Part model, mm, in its own coordinate system. Give positions to 0.01 mm unless a question says otherwise; leave off trailing zeros. Loops run counter-clockwise (first coordinate to the right, second up) from the corner with the lowest first, then second, coordinate; pieces in that order, holes last. Notation, with made-up numbers: (9, 72.25) -> (25, 72.25) arc R22 ccw to (25, 110.25) -> close; hole circle Ø1 at (66, -25.5). An arc over 180 degrees is marked (long way). Write item = value, one per line.
from build123d import *

# Parameters (mm, degrees)
SKETCH1_R           = 1.0922
SKETCH1_R_2         = 2.1
BOSS_EXTRUDE1_DEPTH = 1.5875


with BuildPart() as part:
    # Sketch1 → Boss-Extrude1 (new body)
    with BuildSketch(Plane.XY):
        with BuildLine():
            Line((13.360883802, 35.680481836), (49.041365638, 22.319598034))
            ThreePointArc((49.041365638, 22.319598034), (64.516692787, 0), (49.041365638, -22.319598034))
            Line((49.041365638, -22.319598034), (13.360883802, -35.680481836))
            ThreePointArc((13.360883802, -35.680481836), (-38.1, 0), (13.360883802, 35.680481836))
        make_face()
        with Locations((61.341692787, 0)):
            Circle(SKETCH1_R, mode=Mode.SUBTRACT)
        with Locations((25.4, 27.782025366)):
            Circle(SKETCH1_R, mode=Mode.SUBTRACT)
        with Locations((25.4, -27.782025366)):
            Circle(SKETCH1_R, mode=Mode.SUBTRACT)
        with Locations((-34.925, 0)):
            Circle(SKETCH1_R, mode=Mode.SUBTRACT)
        with Locations((6.35, 0)):
            Circle(SKETCH1_R_2, mode=Mode.SUBTRACT)
        with Locations((-3.175, -5.499261314)):
            Circle(SKETCH1_R_2, mode=Mode.SUBTRACT)
        with Locations((-3.175, 5.499261314)):
            Circle(SKETCH1_R_2, mode=Mode.SUBTRACT)
    extrude(amount=BOSS_EXTRUDE1_DEPTH)


solid = part.part
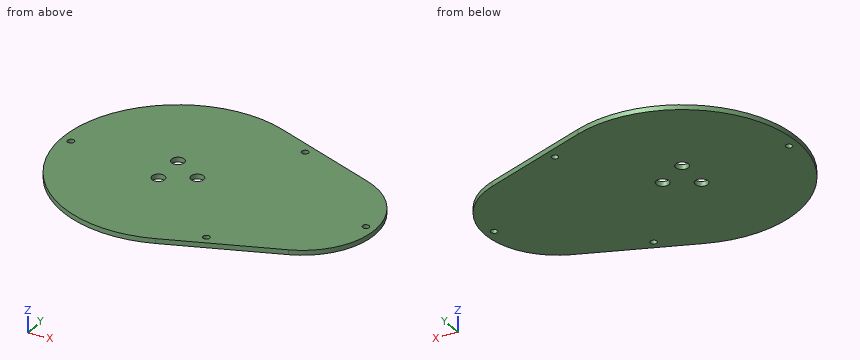
1) Slice it at C-C, the plane z = 0.9. List the corners of the cut face in (x, y) (3 decimals), and give its area (3 significant figures).
Resolved:
outline = (13.361, -35.68) -> (49.041, -22.32) arc R23.833 ccw to (49.041, 22.32) -> (13.361, 35.68) arc R38.1 ccw (long way) to start; hole circle Ø2.184 at (-34.925, 0); hole circle Ø4.2 at (-3.175, -5.499); hole circle Ø4.2 at (-3.175, 5.499); hole circle Ø4.2 at (6.35, 0); hole circle Ø2.184 at (25.4, -27.782); hole circle Ø2.184 at (25.4, 27.782); hole circle Ø2.184 at (61.342, 0)
area = 5,790 mm²
2) Slice it at D-D, the plane x = 6.35. List the corners of the cut face in (y, z).
Resolved:
outline = (-37.57, 0) -> (-2.1, 0) -> (-2.1, 1.59) -> (-37.57, 1.59) -> close; (2.1, 0) -> (37.57, 0) -> (37.57, 1.59) -> (2.1, 1.59) -> close
3) Slice it at A-A, the plane y = 0. List the corners of the cut face in (x, z).
Resolved:
outline = (-38.1, 0) -> (-36.02, 0) -> (-36.02, 1.59) -> (-38.1, 1.59) -> close; (-33.83, 0) -> (4.25, 0) -> (4.25, 1.59) -> (-33.83, 1.59) -> close; (8.45, 0) -> (60.25, 0) -> (60.25, 1.59) -> (8.45, 1.59) -> close; (62.43, 0) -> (64.52, 0) -> (64.52, 1.59) -> (62.43, 1.59) -> close
4) Slice it at B-B, the plane x = 25.4. List the corners of the cut face in (y, z).
Resolved:
outline = (-31.17, 0) -> (-28.87, 0) -> (-28.87, 1.59) -> (-31.17, 1.59) -> close; (-26.69, 0) -> (26.69, 0) -> (26.69, 1.59) -> (-26.69, 1.59) -> close; (28.87, 0) -> (31.17, 0) -> (31.17, 1.59) -> (28.87, 1.59) -> close
5) Drill centre lines: line 1 along Y through (x, z) = (25, 1.45); line 2 along Y through (x, z) = (25.4, 0.65); line 3 along X through (y, z) = (5, 0.65). Where is each one in solid material? Low to high. Write a range as [from, to].
Resolved:
line_1 = [-31.32, -28.8], [-26.77, 26.77], [28.8, 31.32]
line_2 = [-31.17, -28.87], [-26.69, 26.69], [28.87, 31.17]
line_3 = [-37.77, -5.21], [-1.14, 63.99]
